Check sheet for the drawn part. Datum: minimum x, y, z corner. Units: mm. A direction names the side the tool comes from. Give positions to 0.01 mm unless a question says otherwise; leave off trailing zeros. Write each loop counter-clockwise with the first axis right and the second up, starting at its lowest first coordinate (ties: lowest second). Pieces come first, ordered by that corner, then holes. Notation, with made-up numbers: (43, 49.5) - (89, 49.5) arc R18 ccw to (89, 54.5) - close; hole circle Ø10 at (48.5, -23). An arc over 180 degrees is marked (long way). Answer as a JSON object with one key per item and string values. Group by question number.
Item 1: Tool access check on the marked faces 1, 2, 3, 4 and 5. Record the directions out of +Z, -Z, +X, -X, +Y, -Y that give a thin tool (end or side, any length) a straight path to the whole face; none if there is none.
Item 2: Sectioned sample at C-C, the plane y = 205. Record the boundary of the cut face in (x, z).
Item 3: Sectioned sample at D-D, the plane x = 93. Record the boundary of the cut face in (y, z) (1 decimal).
Item 4: Scan lines: line 1 along X through (y, z) = (260, 12); line 2 along Y through (x, z) = (145, 21.5); line 3 along Y through (x, z) = (144, 47) (1 decimal). Record each from-to range of solid material in increasing order. Write a range as [from, to].
Item 5: Sectioned sample at B-B, the plane y = 30. Record the boundary of the cut face in (x, z).
Item 6: Sectioned sample at A-A, the plane x = 145. Record the boundary of the cut face in (y, z).
Item 7: Go/stop test with flat-tipped pins: pin 1 (12 mm diameter, centred on x = 134.5, y = 124.5, fed in from +Z); pin 2 (5 mm diameter, centred on x = 105, z = 92, fed in from +Y); pin 3 (20 mm diameter, centred on y = 125, z = 82, fed in from +X). Record where each tip stops, or that it passes through.
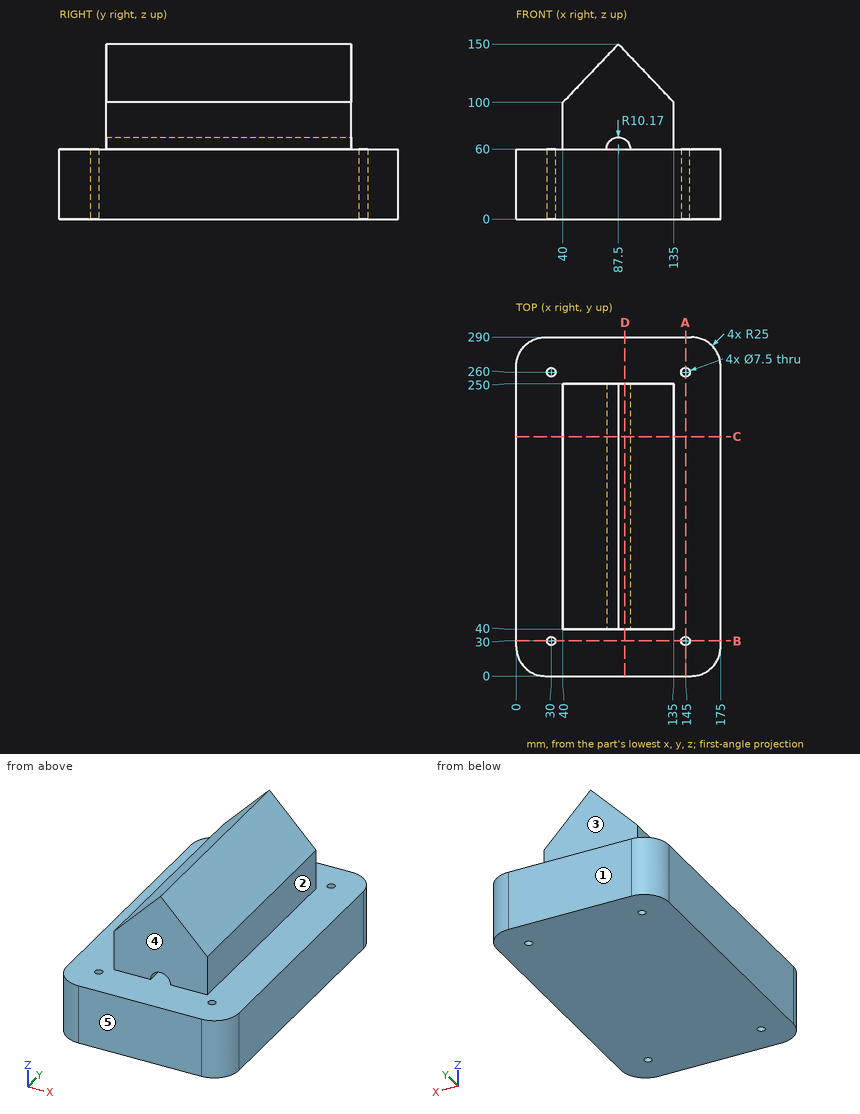
Geometry check:
{
 "1": {"face 1": "+Z, -Z, +X, -X, +Y", "face 2": "+Z, +X, +Y, -Y", "face 3": "+Z, +X, -X, +Y", "face 4": "+Z, +X, -X, -Y", "face 5": "+Z, -Z, +X, -X, -Y"},
 "2": {"outline": "(0, 0) - (175, 0) - (175, 60) - (135, 60) - (135, 100) - (87.5, 150) - (40, 100) - (40, 60) - (0, 60) - close; hole (77.33, 60) - (97.67, 60) arc R10.17 ccw to start"},
 "3": {"outline": "(0, 0) - (290, 0) - (290, 60) - (0, 60) - close; (40, 68.6) - (250, 68.6) - (250, 144.2) - (40, 144.2) - close"},
 "4": {"line 1": "[0, 26.25], [33.75, 141.25], [148.75, 175]", "line 2": "[0, 26.25], [33.75, 256.25], [263.75, 290]", "line 3": "[0, 26.4], [33.6, 256.4], [263.6, 290]"},
 "5": {"outline": "(0, 0) - (26.25, 0) - (26.25, 60) - (0, 60) - close; (33.75, 0) - (141.25, 0) - (141.25, 60) - (33.75, 60) - close; (148.75, 0) - (175, 0) - (175, 60) - (148.75, 60) - close"},
 "6": {"outline": "(0, 0) - (26.25, 0) - (26.25, 60) - (0, 60) - close; (33.75, 0) - (256.25, 0) - (256.25, 60) - (33.75, 60) - close; (263.75, 0) - (290, 0) - (290, 60) - (263.75, 60) - close"},
 "7": {"pin 1": "z = 106.84", "pin 2": "y = 250", "pin 3": "x = 135"}
}
